Geometry: final body of the model. Coordinates: model frame, mm. A direction names the side the tool comes from. Round coordinates to 2 decimals unless told otherwise and drop trailing zeros. Write each loop counter-clockwise with the first axis right and the second up, starting at its lowest first coordinate (ties: lowest second). Pieces come first, ordered by that corner, then holes. Notation, with made-up numbers: (27.25, 16) -> (63.25, 16) arc R30 ccw to (63.25, 47) -> close; hole circle Ø9 at (-11.5, 81). An arc over 180 degrees is marked (long way). Use one line per item in the form item = value. Start each with the question number.
1. Cut plane D-D, the plane x = -1.95. Return the cut outline in (y, z).
2. Reachability of faces 4 (the face through (0, 2, 2.9)), 5 (the face through (0, -1, -0.3)), 6 (the face through (-6.35, 5, 0)), 7 (the face through (-2, 7, -1.45)), 8 (the face through (6.35, 5, 0)) from +Z, -Z, +X, -X, +Y, -Y: full face, straight path, thin tool, end or side. Return the list, or none.
3. Draft query along X for faces 1 (the face through (6.4, 2, 0)), 2 (the face through (2.46, 0.89, 0.04)), 3 (the face through (0, 5, 2.95)). Return one class per face: pulls with the +X half, pulls with the -X half, needs draft (parallel to the pull), parting line crosses it, or undercut.
4. Cut plane B-B, the plane x = 3.25. Return the cut outline in (y, z).
5. Cut plane C-C, the plane z = -0.45. Return the cut outline in (x, y).
6. Line query: L1, parallel to Y at x = -3.25, z = 1.3; L2, parallel to Y at x = 3.25, z = 0.35; L3, parallel to Y at x = -0.75, z = 1.3. Output: solid intervals per line, ascending.
7. Pin query (flat end, axial travel): pin 1 Ø0.7 at (x, y) = (-2, 7) entering from -Z; pin 2 Ø0.5 at (y, z) = (-2, 0) entering from +X; pin 3 Ø0.5 at (y, z) = (-1.5, 0) entering from -X; pin 4 Ø2 at (x, z) = (-5, -0.5) entering from -Y. Return the tip coordinate at first contact, or that it passes through.
8. Cut plane A-A, the plane y = -1.5. Return the cut outline in (x, z), plus the area to 3 significant figures.
```python
from build123d import *
from OCP.BRepFilletAPI import BRepFilletAPI_MakeChamfer

# Parameters (mm, degrees)
SKETCH1_W                = 12.8
SKETCH1_H                = 5.8
BOSS_EXTRUDE1_DEPTH      = 3.5
SKETCH2_W                = 0.9
SKETCH2_H                = 0.6
BOSS_EXTRUDE3_DEPTH      = 3.5
CHAMFER1_SIZE            = 0.5
CHAMFER1_SIZE2           = 0.133974596
SKETCH3_R                = 1.1
SKETCH3_R_2              = 1
CUT_EXTRUDE1_DEPTH       = 5.8
SKETCH4_W                = 12.7
SKETCH4_H                = 5.9
BOSS_EXTRUDE4_DEPTH      = 3
BOSS_EXTRUDE5_DEPTH      = 1.45
BOSS_EXTRUDE5_DEPTH_BACK = 1.45
SKETCH6_W                = 0.3
SKETCH6_H                = 4.08
CUT_EXTRUDE2_DEPTH       = 0.4


with BuildPart() as part:
    # Sketch1 → Boss-Extrude1 (new body)
    with BuildSketch(Plane(origin=(0, 0, 0), x_dir=(1, 0, 0), z_dir=(0, 1, 0))):
        Rectangle(SKETCH1_W, SKETCH1_H)
    extrude(amount=BOSS_EXTRUDE1_DEPTH)

    # Sketch2 → Boss-Extrude3 (add)
    with BuildSketch(Plane.XZ):
        Rectangle(SKETCH2_W, SKETCH2_H)
        with Locations((-5.08, 0)):
            Rectangle(SKETCH2_W, SKETCH2_H)
        with Locations((5.08, 0)):
            Rectangle(SKETCH2_W, SKETCH2_H)
    extrude(amount=BOSS_EXTRUDE3_DEPTH)

    # Chamfer1: one chamfer whose edges measure the first distance from different faces: ONE call of the kernel's chamfer builder (chamfer() names one face for all edges)
    chamfer1_edges_1 = [part.edges().sort_by_distance(p)[0] for p in [
        (0.45, -3.5, 0),
    ]]
    chamfer1_side_1 = [part.faces().sort_by_distance(p)[0] for p in [
        (0.45, -1.75, 0),
    ]]
    chamfer1_edges_2 = [part.edges().sort_by_distance(p)[0] for p in [
        (0, -3.5, 0.3),
    ]]
    chamfer1_side_2 = [part.faces().sort_by_distance(p)[0] for p in [
        (0, -1.75, 0.3),
    ]]
    chamfer1_edges_3 = [part.edges().sort_by_distance(p)[0] for p in [
        (-0.45, -3.5, 0),
    ]]
    chamfer1_side_3 = [part.faces().sort_by_distance(p)[0] for p in [
        (-0.45, -1.75, 0),
    ]]
    chamfer1_edges_4 = [part.edges().sort_by_distance(p)[0] for p in [
        (0, -3.5, -0.3),
    ]]
    chamfer1_side_4 = [part.faces().sort_by_distance(p)[0] for p in [
        (0, -1.75, -0.3),
    ]]
    chamfer1_edges_5 = [part.edges().sort_by_distance(p)[0] for p in [
        (-4.63, -3.5, 0),
    ]]
    chamfer1_side_5 = [part.faces().sort_by_distance(p)[0] for p in [
        (-4.63, -1.75, 0),
    ]]
    chamfer1_edges_6 = [part.edges().sort_by_distance(p)[0] for p in [
        (-5.08, -3.5, 0.3),
    ]]
    chamfer1_side_6 = [part.faces().sort_by_distance(p)[0] for p in [
        (-5.08, -1.75, 0.3),
    ]]
    chamfer1_edges_7 = [part.edges().sort_by_distance(p)[0] for p in [
        (-5.53, -3.5, 0),
    ]]
    chamfer1_side_7 = [part.faces().sort_by_distance(p)[0] for p in [
        (-5.53, -1.75, 0),
    ]]
    chamfer1_edges_8 = [part.edges().sort_by_distance(p)[0] for p in [
        (-5.08, -3.5, -0.3),
    ]]
    chamfer1_side_8 = [part.faces().sort_by_distance(p)[0] for p in [
        (-5.08, -1.75, -0.3),
    ]]
    chamfer1_edges_9 = [part.edges().sort_by_distance(p)[0] for p in [
        (5.53, -3.5, 0),
    ]]
    chamfer1_side_9 = [part.faces().sort_by_distance(p)[0] for p in [
        (5.53, -1.75, 0),
    ]]
    chamfer1_edges_10 = [part.edges().sort_by_distance(p)[0] for p in [
        (5.08, -3.5, 0.3),
    ]]
    chamfer1_side_10 = [part.faces().sort_by_distance(p)[0] for p in [
        (5.08, -1.75, 0.3),
    ]]
    chamfer1_edges_11 = [part.edges().sort_by_distance(p)[0] for p in [
        (4.63, -3.5, 0),
    ]]
    chamfer1_side_11 = [part.faces().sort_by_distance(p)[0] for p in [
        (4.63, -1.75, 0),
    ]]
    chamfer1_edges_12 = [part.edges().sort_by_distance(p)[0] for p in [
        (5.08, -3.5, -0.3),
    ]]
    chamfer1_side_12 = [part.faces().sort_by_distance(p)[0] for p in [
        (5.08, -1.75, -0.3),
    ]]
    chamfer1 = BRepFilletAPI_MakeChamfer(part.part.solid().wrapped)
    for e in chamfer1_edges_1:
        chamfer1.Add(CHAMFER1_SIZE, CHAMFER1_SIZE2, e.wrapped, chamfer1_side_1[0].wrapped)  # the first distance lies on this face
    for e in chamfer1_edges_2:
        chamfer1.Add(CHAMFER1_SIZE, CHAMFER1_SIZE2, e.wrapped, chamfer1_side_2[0].wrapped)  # the first distance lies on this face
    for e in chamfer1_edges_3:
        chamfer1.Add(CHAMFER1_SIZE, CHAMFER1_SIZE2, e.wrapped, chamfer1_side_3[0].wrapped)  # the first distance lies on this face
    for e in chamfer1_edges_4:
        chamfer1.Add(CHAMFER1_SIZE, CHAMFER1_SIZE2, e.wrapped, chamfer1_side_4[0].wrapped)  # the first distance lies on this face
    for e in chamfer1_edges_5:
        chamfer1.Add(CHAMFER1_SIZE, CHAMFER1_SIZE2, e.wrapped, chamfer1_side_5[0].wrapped)  # the first distance lies on this face
    for e in chamfer1_edges_6:
        chamfer1.Add(CHAMFER1_SIZE, CHAMFER1_SIZE2, e.wrapped, chamfer1_side_6[0].wrapped)  # the first distance lies on this face
    for e in chamfer1_edges_7:
        chamfer1.Add(CHAMFER1_SIZE, CHAMFER1_SIZE2, e.wrapped, chamfer1_side_7[0].wrapped)  # the first distance lies on this face
    for e in chamfer1_edges_8:
        chamfer1.Add(CHAMFER1_SIZE, CHAMFER1_SIZE2, e.wrapped, chamfer1_side_8[0].wrapped)  # the first distance lies on this face
    for e in chamfer1_edges_9:
        chamfer1.Add(CHAMFER1_SIZE, CHAMFER1_SIZE2, e.wrapped, chamfer1_side_9[0].wrapped)  # the first distance lies on this face
    for e in chamfer1_edges_10:
        chamfer1.Add(CHAMFER1_SIZE, CHAMFER1_SIZE2, e.wrapped, chamfer1_side_10[0].wrapped)  # the first distance lies on this face
    for e in chamfer1_edges_11:
        chamfer1.Add(CHAMFER1_SIZE, CHAMFER1_SIZE2, e.wrapped, chamfer1_side_11[0].wrapped)  # the first distance lies on this face
    for e in chamfer1_edges_12:
        chamfer1.Add(CHAMFER1_SIZE, CHAMFER1_SIZE2, e.wrapped, chamfer1_side_12[0].wrapped)  # the first distance lies on this face
    add(Compound.cast(chamfer1.Shape()), mode=Mode.REPLACE)

    # Sketch3 → Cut-Extrude1 (cut)
    with BuildSketch(Plane.XY.offset(2.9)):
        with Locations((-3.25, 1.5)):
            Circle(SKETCH3_R)
        with Locations((3.25, 1.5)):
            Circle(SKETCH3_R_2)
    extrude(amount=-CUT_EXTRUDE1_DEPTH, mode=Mode.SUBTRACT)

    # Sketch4 → Boss-Extrude4 (add)
    with BuildSketch(Plane(origin=(0, 3.5, 0), x_dir=(1, 0, 0), z_dir=(0, 1, 0))):
        Rectangle(SKETCH4_W, SKETCH4_H)
    extrude(amount=BOSS_EXTRUDE4_DEPTH)

    # Sketch5 → Boss-Extrude5 (add, two sides: drawn at the far end of the back side and taken through both)
    with BuildSketch(Plane.XY.offset(-BOSS_EXTRUDE5_DEPTH_BACK)):
        with BuildLine():
            Line((-2.55, 6.5), (-2.55, 6.75))
            ThreePointArc((-2.55, 6.75), (-1.95, 7.35), (-1.35, 6.75))
            Line((-1.35, 6.75), (-1.35, 6.5))
            Line((-1.35, 6.5), (-2.55, 6.5))
        make_face()
    extrude(amount=BOSS_EXTRUDE5_DEPTH + BOSS_EXTRUDE5_DEPTH_BACK)

    # Sketch6 → Cut-Extrude2 (cut)
    with BuildSketch(Plane(origin=(0, 6.5, 0), x_dir=(1, 0, 0), z_dir=(0, 1, 0))):
        with Locations((-5.5, 0)):
            Rectangle(SKETCH6_W, SKETCH6_H)
    extrude(amount=-CUT_EXTRUDE2_DEPTH, mode=Mode.SUBTRACT)


solid = part.part
```
Outcome:
q1.outline = (0, -2.9) -> (3.5, -2.9) -> (3.5, -2.95) -> (6.5, -2.95) -> (6.5, -1.45) -> (7.35, -1.45) -> (7.35, 1.45) -> (6.5, 1.45) -> (6.5, 2.95) -> (3.5, 2.95) -> (3.5, 2.9) -> (0, 2.9) -> close
q2.face_4 = +Z, +X, -X, -Y
q2.face_5 = -Z, +X, -X, -Y
q2.face_6 = +Z, -Z, -X, +Y
q2.face_7 = -Z, +X, -X, +Y
q2.face_8 = +Z, -Z, +X, +Y
q3.face_1 = pulls with the +X half
q3.face_2 = undercut
q3.face_3 = needs draft
q4.outline = (0, -2.9) -> (0.5, -2.9) -> (0.5, 2.9) -> (0, 2.9) -> close; (2.5, -2.9) -> (3.5, -2.9) -> (3.5, -2.95) -> (6.5, -2.95) -> (6.5, 2.95) -> (3.5, 2.95) -> (3.5, 2.9) -> (2.5, 2.9) -> close
q5.outline = (-6.4, 0) -> (6.4, 0) -> (6.4, 3.5) -> (6.35, 3.5) -> (6.35, 6.5) -> (-1.35, 6.5) -> (-1.35, 6.75) arc R0.6 ccw to (-2.55, 6.75) -> (-2.55, 6.5) -> (-5.35, 6.5) -> (-5.35, 6.1) -> (-5.65, 6.1) -> (-5.65, 6.5) -> (-6.35, 6.5) -> (-6.35, 3.5) -> (-6.4, 3.5) -> close; hole circle Ø2.2 at (-3.25, 1.5); hole circle Ø2 at (3.25, 1.5)
q6.L1 = 0 to 0.4, 2.6 to 6.5
q6.L2 = 0 to 0.5, 2.5 to 6.5
q6.L3 = 0 to 6.5
q7.pin_1 = -1.45
q7.pin_2 = 5.53
q7.pin_3 = -5.53
q7.pin_4 = -3.5
q8.outline = (-5.53, -0.3) -> (-4.63, -0.3) -> (-4.63, 0.3) -> (-5.53, 0.3) -> close; (-0.45, -0.3) -> (0.45, -0.3) -> (0.45, 0.3) -> (-0.45, 0.3) -> close; (4.63, -0.3) -> (5.53, -0.3) -> (5.53, 0.3) -> (4.63, 0.3) -> close
q8.area = 1.62 mm^2
